Here's the drawing with two shaded views (mm, measured from the low corner). I have some questions. Round coordinates to 2 decimals unless told otherwise and drop trailing zeros. Loops run counter-clockwise (first coordinate to the right, second up) from the corner with the lowest first, then second, coordinate; pieces in that order, holes last.
(1) I want a section at B-B on y = 9. Write out the boundary of the cut face in (x, z).
(2) Thinking about a two-plate mould opening in X: for the marked faces 1 and 2, which applies, released by +X, released by -X, zero draft, split by the parting line, or undercut?
(3) If I drill on line 1 along X through (y, z) = (10, 1.1); line 2 along Y through (x, z) = (8, 1.2), over which ranges is the centre line in solid material (lowest first)?
(4) Will these pins go through, and if not, where does the flat tip stop? pin 1 Ø0.6 at (y, z) = (6.5, 1) entering from -X; pin 2 Ø0.5 at (x, y) = (7.5, 6.5) entering from +Z.
(5) I want a section at A-A on z = 1.3. Write out the boundary of the cut face in (x, y).
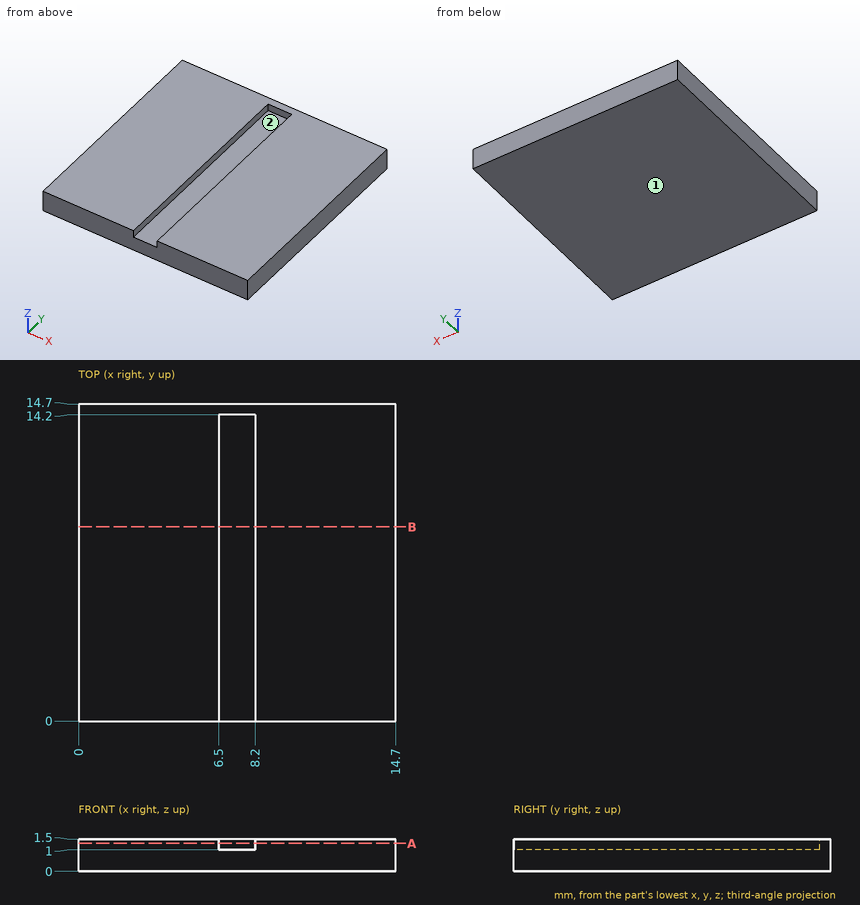
Filled sheet:
1. outline: (0, 0) - (14.7, 0) - (14.7, 1.5) - (8.2, 1.5) - (8.2, 1) - (6.5, 1) - (6.5, 1.5) - (0, 1.5) - close
2. face 1: zero draft
2. face 2: undercut
3. line 1: x = 0 to 6.5, 8.2 to 14.7
3. line 2: y = 14.2 to 14.7
4. pin 1: stops at x = 0
4. pin 2: stops at z = 1
5. outline: (0, 0) - (6.5, 0) - (6.5, 14.2) - (8.2, 14.2) - (8.2, 0) - (14.7, 0) - (14.7, 14.7) - (0, 14.7) - close
